from build123d import *

# Parameters (mm, degrees)
F0_W     = 940
F0_H     = 2
F0_W_2   = 2
F0_H_2   = 28
F0_W_3   = 28
F1_DEPTH = 40
F0_H_3   = 740
F2_DEPTH = 2


with BuildPart() as f1:
    # F0 (on Top) → F1 (new body)
    with BuildSketch(Plane.XY):
        Polygon((119.6999707818, 869.6999302506), (121.6999707818, 869.6999302506), (121.6999707818, 897.6999302506), (149.6999707818, 897.6999302506), (149.6999707818, 899.6999302506), (119.6999707818, 899.6999302506), align=None)
        with Locations((619.6999707818, 898.6999302506)):
            Rectangle(F0_W, F0_H)
        Polygon((119.6999707818, 179.6999302506), (119.6999707818, 129.6999302506), (121.6999707818, 129.6999302506), (121.6999707818, 869.6999302506), (119.6999707818, 869.6999302506), align=None)
        Polygon((1117.6999707818, 897.6999302506), (1117.6999707818, 869.6999302506), (1119.6999707818, 869.6999302506), (1119.6999707818, 899.6999302506), (1089.6999707818, 899.6999302506), (1089.6999707818, 897.6999302506), align=None)
        Polygon((1117.6999707818, 869.6999302506), (1117.6999707818, 129.6999302506), (1119.6999707818, 129.6999302506), (1119.6999707818, 179.6999302506), (1119.6999707818, 869.6999302506), align=None)
        with Locations((1118.6999707818, 115.6999302506)):
            Rectangle(F0_W_2, F0_H_2)
        with Locations((1118.6999707818, 100.6999302506)):
            Rectangle(F0_W_2, F0_H)
        with Locations((1103.6999707818, 100.6999302506)):
            Rectangle(F0_W_3, F0_H)
        with Locations((619.6999707818, 100.6999302506)):
            Rectangle(F0_W, F0_H)
        with Locations((135.6999707818, 100.6999302506)):
            Rectangle(F0_W_3, F0_H)
        with Locations((120.6999707818, 100.6999302506)):
            Rectangle(F0_W_2, F0_H)
        with Locations((120.6999707818, 115.6999302506)):
            Rectangle(F0_W_2, F0_H_2)
    extrude(amount=-F1_DEPTH)

    # F0 (on Top) → F2 (join)
    with BuildSketch(Plane.XY):
        Polygon((121.6999707818, 129.6999302506), (121.6999707818, 101.6999302506), (149.6999707818, 101.6999302506), (1089.6999707818, 101.6999302506), (1117.6999707818, 101.6999302506), (1117.6999707818, 129.6999302506), (1117.6999707818, 869.6999302506), (1117.6999707818, 897.6999302506), (1089.6999707818, 897.6999302506), (149.6999707818, 897.6999302506), (121.6999707818, 897.6999302506), (121.6999707818, 869.6999302506), align=None)
        with Locations((619.6999707818, 499.6999302506)):
            Rectangle(F0_W, F0_H_3, mode=Mode.SUBTRACT)
    extrude(amount=-F2_DEPTH)


solid = f1.part
Build history of the part. All positions in model axes, mm. A direction names the side the tool comes from. Coordinates: 2 decimals unless noted, no trailing zeros. Write each loop counter-clockwise with the first axis right and the second up, starting at its lowest first coordinate (ties: lowest second). Pieces come first, ordered by that corner, then holes.
(1) Cut at A-A on y = 203. List the corners of the cut face in (x, z), and give its area (3 significant figures).
(2) Cut at B-B on z = -18.5. List the corners of the cut face in (x, y).
(3) 3-axis set-ups, long thin cutter, end or side, ignore diameter. For faces 1 (the flat face through (1117.7, 505, -21)), 2 (the flat face through (580, 116, 0)): which of +Z, -Z, +X, -X, +Y, -Y reach the whole face in a straight line?
(4) Mould opens along Y. For faces 3 (the flat face through (613, 99.7, -20)), 4 (the flat face through (613, 897.7, -21)), 5 (the flat face through (119.7, 505, -20)) say: pulls with the +Y half, pulls with the -Y half, needs draft (parallel to the pull), parting line crosses it, or undercut.
(5) Cut at C-C on x = 288.5. List the corners of the cut face in (y, z), and give its area (3 significant figures).
(6) Drill centre lines: line 1 (Y direction, x = 223.5, z = -8); line 2 (X direction, y = 592.5, z = -24). Where is each one in solid material? Low to high.
Working result:
1. outline: (119.7, -40) - (121.7, -40) - (121.7, -2) - (149.7, -2) - (149.7, 0) - (119.7, 0) - close; (1089.7, -2) - (1117.7, -2) - (1117.7, -40) - (1119.7, -40) - (1119.7, 0) - (1089.7, 0) - close
1. area: 272 mm2
2. outline: (119.7, 99.7) - (1119.7, 99.7) - (1119.7, 899.7) - (119.7, 899.7) - close; hole (121.7, 101.7) - (1117.7, 101.7) - (1117.7, 897.7) - (121.7, 897.7) - close
3. face 1: -Z
3. face 2: +Z, +X, -X, +Y, -Y
4. face 3: pulls with the -Y half
4. face 4: undercut
4. face 5: needs draft
5. outline: (99.7, -40) - (101.7, -40) - (101.7, -2) - (129.7, -2) - (129.7, 0) - (99.7, 0) - close; (869.7, -2) - (897.7, -2) - (897.7, -40) - (899.7, -40) - (899.7, 0) - (869.7, 0) - close
5. area: 272 mm2
6. line 1: y = 99.7 to 101.7, 897.7 to 899.7
6. line 2: x = 119.7 to 121.7, 1117.7 to 1119.7
